Part model, mm, in its own coordinate system. Give positions to 0.01 mm unless a question says otherwise; leave off trailing zeros. Order: outer loops, then holes, each group sorted by start corner. A loop starts at its lowest first (then second) coordinate and runs counter-clockwise, first axis right, second up. Notation, with made-up numbers: (67.5, 32.5) - (98.5, 32.5) arc R16 ccw to (98.5, 41.5) - close; hole circle Ø11 at (58, -18). An arc over 180 degrees is marked (long way). One line per item, written item: value.
```python
from build123d import *

# Parameters (mm, degrees)
SKETCH1_R           = 2.5
BOSS_EXTRUDE1_DEPTH = 10
CUT_EXTRUDE1_DEPTH  = 5
SKETCH2_R           = 2.5
SKETCH2_R_2         = 5
CUT_EXTRUDE2_DEPTH  = 241.282833344


with BuildPart() as part:
    # Sketch1 → Boss-Extrude1 (new body)
    with BuildSketch(Plane.XY):
        Polygon((0, 0), (132.8, 0), (132.8, 65), (83.664018374, 200), (0, 200), align=None)
        with Locations((115.1, 27)):
            Circle(SKETCH1_R, mode=Mode.SUBTRACT)
        with Locations((89.1, 27)):
            Circle(SKETCH1_R, mode=Mode.SUBTRACT)
        with Locations((115.1, 53)):
            Circle(SKETCH1_R, mode=Mode.SUBTRACT)
        with Locations((89.1, 53)):
            Circle(SKETCH1_R, mode=Mode.SUBTRACT)
        with Locations((17.7, 53)):
            Circle(SKETCH1_R, mode=Mode.SUBTRACT)
        with Locations((17.7, 27)):
            Circle(SKETCH1_R, mode=Mode.SUBTRACT)
        with Locations((43.7, 27)):
            Circle(SKETCH1_R, mode=Mode.SUBTRACT)
        with Locations((43.7, 53)):
            Circle(SKETCH1_R, mode=Mode.SUBTRACT)
        with Locations((59.91, 29.92)):
            Circle(SKETCH1_R, mode=Mode.SUBTRACT)
        with Locations((59.91, 9.92)):
            Circle(SKETCH1_R, mode=Mode.SUBTRACT)
    extrude(amount=BOSS_EXTRUDE1_DEPTH)

    # Sketch1_3 → Cut-Extrude1 (cut)
    with BuildSketch(Plane.XY):
        Polygon((64.535, 29.92), (62.2225, 33.925367493), (57.5975, 33.925367493), (55.285, 29.92), (57.5975, 25.914632507), (62.2225, 25.914632507), align=None)
        Polygon((62.2225, 13.925367493), (64.535, 9.92), (62.2225, 5.914632507), (57.5975, 5.914632507), (55.285, 9.92), (57.5975, 13.925367493), align=None)
    extrude(amount=CUT_EXTRUDE1_DEPTH, mode=Mode.SUBTRACT)

    # Sketch2 → Cut-Extrude2 (cut, through all)
    with BuildSketch(Plane(origin=(0, 0, 0), x_dir=(-1, 0, 0), z_dir=(0, 0, -1))):
        with Locations((-35, 187.5)):
            Circle(SKETCH2_R)
        with Locations((-15, 187.5)):
            Circle(SKETCH2_R)
        with Locations((-35, 110)):
            Circle(SKETCH2_R)
        with Locations((-15, 110)):
            Circle(SKETCH2_R)
        with Locations((-57, 148.75)):
            Circle(SKETCH2_R_2)
        with Locations((-77, 148.75)):
            Circle(SKETCH2_R)
        with Locations((-37, 148.75)):
            Circle(SKETCH2_R)
    extrude(amount=-CUT_EXTRUDE2_DEPTH, mode=Mode.SUBTRACT)


solid = part.part
```
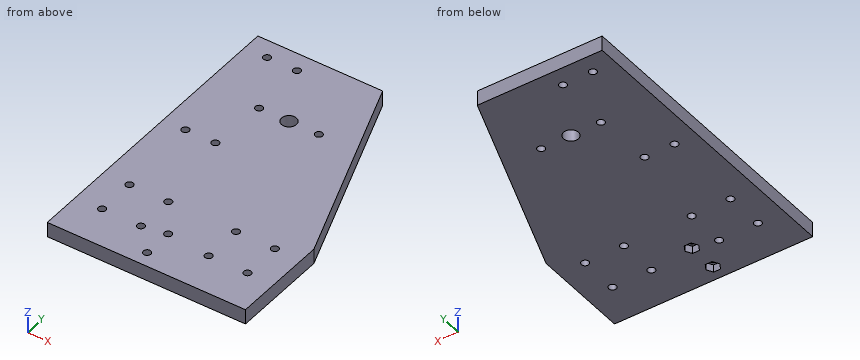
1) Cut at C-C, the plane y = 110. Give the cut face in (x, z), then the cut area to 3 significant figures.
Outcome:
outline: (0, 0) - (12.5, 0) - (12.5, 10) - (0, 10) - close; (17.5, 0) - (32.5, 0) - (32.5, 10) - (17.5, 10) - close; (37.5, 0) - (116.42, 0) - (116.42, 10) - (37.5, 10) - close
area: 1,060 mm^2
2) Cut at B-B, the plane z = 8.25. Give the number of separate pieces and of enclosed holes in the cut face, then the cut area to 3 significant figures.
Outcome:
separate pieces: 1
enclosed holes: 17
area: 22,900 mm^2
3) Cut at A-A, the plane x = 43.7. Give the cut face in (y, z), then the cut area to 3 significant figures.
Outcome:
outline: (0, 0) - (24.5, 0) - (24.5, 10) - (0, 10) - close; (29.5, 0) - (50.5, 0) - (50.5, 10) - (29.5, 10) - close; (55.5, 0) - (200, 0) - (200, 10) - (55.5, 10) - close
area: 1,900 mm^2
4) Drill centre lines: line 1 along Y through (x, z) = (37, 5.75); line 2 along X through (y, z) = (9.92, 6.9); line 3 along Y through (x, z) = (60, 2). Where is each one in solid material? Low to high. Write a range as from..to.
Outcome:
line 1: y = 0..108.5, 111.5..146.25, 151.25..186, 189..200
line 2: x = 0..57.41, 62.41..132.8
line 3: y = 0..5.91, 13.93..25.91, 33.93..144.75, 152.75..200
5) Pin check, flat tips, straight feed: pin 1 (4.5 mm diameter, centred on x = 43.7, y = 27, fed in from -Z); pin 2 (2.5 mm diameter, centred on x = 60.5, y = 8.5, fed in from -Z); pin 3 (5 mm diameter, centred on y = 110, z = 3.5, fed in from +X); pin 4 (5 mm diameter, centred on y = 179, z = 8.5, fed in from +X). Stop position of each tip, or through.
Outcome:
pin 1: passes through
pin 2: stops at z = 5
pin 3: stops at x = 117.33
pin 4: stops at x = 92.22
6) Cut at D-D, the plane x = 59.91. Give the cut face in (y, z), then the cut area to 3 significant figures.
Outcome:
outline: (0, 0) - (5.91, 0) - (5.91, 5) - (7.42, 5) - (7.42, 10) - (0, 10) - close; (12.42, 5) - (13.93, 5) - (13.93, 0) - (25.91, 0) - (25.91, 5) - (27.42, 5) - (27.42, 10) - (12.42, 10) - close; (32.42, 5) - (33.93, 5) - (33.93, 0) - (144.68, 0) - (144.68, 10) - (32.42, 10) - close; (152.82, 0) - (200, 0) - (200, 10) - (152.82, 10) - close
area: 1,790 mm^2
